Autodesk Inventor part; units mm, degrees
ref_plane "YZ Plane" through (0, 0, 0) normal (1, 0, 0) x (0, 1, 0)
ref_plane "XZ Plane" through (0, 0, 0) normal (0, 1, 0) x (-1, 0, 0)
ref_plane "XY Plane" through (0, 0, 0) normal (0, 0, 1) x (1, 0, 0)
sketch "Sketch1" plane through (0, 0, 0) normal (0, 1, 0) x (-1, 0, 0)
  line L0 (0, 0) -> (-25.4, 0)
  line L1 (-25.4, 0) -> (-25.4, -25.4)
  line L2 (-25.4, -25.4) -> (0, -25.4)
  line L3 (0, -25.4) -> (0, 0)
  line L4 (-23.8125, -23.8125) -> (-23.8125, -1.5875)
  line L5 (-23.8125, -1.5875) -> (-1.5875, -1.5875)
  line L6 (-1.5875, -1.5875) -> (-1.5875, -23.8125)
  line L7 (-1.5875, -23.8125) -> (-23.8125, -23.8125)
  dimension "d0" = 25.4
  dimension "d1" = 25.4
  dimension "d2" = 1.5875
extrude "Extrusion1" add sketch "Sketch1" along normal blind 238.0191
sketch "Sketch2" plane through (25.4, 0, 0) normal (1, 0, 0) x (0, 0, -1)
  line L0 (0, 0) -> (0, 238.0191)
  line L1 (0, 0) -> (25.4, 26.3769)
  line L2 (25.4, 0) -> (25.4, 238.0191)
  line L3 (0, 0) -> (25.4, 0)
  line L4 (25.4, 26.3769) -> (25.4, 0)
  line L5 (25.4, 0) -> (0, 0)
  dimension "d5" = 43.919
extrude "Extrusion2" cut sketch "Sketch2" against normal blind 25.4
properties part number "frontrollcage" material "Aluminum 6061"
Work out the finished part from the listing and answer in its coordinate system (mm). A direction names the side the tool comes from. Round coordinates to 2 decimals unless told otherwise and drop trailing zeros. Loops run counter-clockwise (first coordinate to the right, second up) from the corner with the lowest first, then second, coordinate; pieces in that order, holes last. Notation, with made-up numbers: (15.5, 63.5) - (40.5, 63.5) arc R11 cw to (40.5, 80.5) - close; hole circle Ø3 at (63, -17.5). An arc over 180 degrees is marked (long way). Use one line per item in the form item = value. Start each with the question number.
(1) Consider line 1 (Z direction, x = 11.75, y = 132); line 2 (X direction, y = 97, z = -11); line 3 (Y direction, x = 15.5, z = -24). Determine where each line is inside the solid, lowest interval first.
(2) Which of the six approach directions +Z, -Z, +X, -X, +Y, -Y give full straight-line access (tool end or side, diameter ignored) to faces 1 (the face through (13, 118, -1.588)), 2 (the face through (13, 131, -25.4))?
(3) Find section B-B on y = 58.5. Determine the outline of the cut face in (x, z).
(4) Find section A-A on x = 19. Determine the outline of the cut face in (y, z).
(5) Determine the mould class of faces 3 (the face through (23.812, 118, -13)), 4 (the face through (1.588, 118, -13)), 5 (the face through (13, 117, 0)), 6 (the face through (0, 117, -13)) for opening direction Z: +Z half, -Z half, draft (parallel to the pull), parting line (faces both ways), or undercut.
(6) Find section C-C on z = -15.75. Determine the outline of the cut face in (x, y), and give its area (3 significant figures).
Answer list:
q1.line_1 = -25.4 to -23.81, -1.59 to 0
q1.line_2 = 0 to 1.59, 23.81 to 25.4
q1.line_3 = 24.92 to 238.02
q2.face_1 = +Y, -Y
q2.face_2 = -Z, +X, -X, +Y, -Y
q3.outline = (0, -25.4) - (25.4, -25.4) - (25.4, 0) - (0, 0) - close; hole (1.59, -23.81) - (23.81, -23.81) - (23.81, -1.59) - (1.59, -1.59) - close
q4.outline = (0, 0) - (1.65, -1.59) - (238.02, -1.59) - (238.02, 0) - close; (24.73, -23.81) - (26.38, -25.4) - (238.02, -25.4) - (238.02, -23.81) - close
q5.face_3 = undercut
q5.face_4 = undercut
q5.face_5 = +Z half
q5.face_6 = draft
q6.outline = (0, 16.36) - (1.59, 16.36) - (1.59, 238.02) - (0, 238.02) - close; (23.81, 16.36) - (25.4, 16.36) - (25.4, 238.02) - (23.81, 238.02) - close
q6.area = 704 mm^2
